from build123d import *

# Parameters (mm, degrees)
BOSS_EXTRU_1_DEPTH       = 320
BOSS_EXTRU_1_DEPTH_BACK  = 10
ESQUISSE3_W              = 200
ESQUISSE3_H              = 6
BOSS_EXTRU_2_DEPTH       = 56.1
ESQUISSE41_W             = 200
ESQUISSE41_H             = 330
BOSS_EXTRU_9_DEPTH       = 3
ENL_V_MAT_EXTRU_22_DEPTH = 6
CONG_8_R                 = 10
CONG_9_R                 = 16
ESQUISSE48_W             = 3
ESQUISSE48_H             = 2.4


with BuildPart() as part:
    # Esquisse1 → Boss.-Extru.1 (new body, two sides)
    with BuildSketch(Plane.XY) as boss_extru_1_sk:
        with BuildLine():
            Line((-95, 2), (95, 2))
            ThreePointArc((95, 2), (97.121320344, 2.878679656), (98, 5))
            Line((98, 5), (98, 17))
            ThreePointArc((98, 17), (99.464466094, 20.535533906), (103, 22))
            Line((103, 22), (127, 22))
            Line((127, 22), (132, 22))
            Line((132, 22), (132, 20))
            Line((132, 20), (127, 20))
            Line((127, 20), (103, 20))
            ThreePointArc((103, 20), (100.878679656, 19.121320344), (100, 17))
            Line((100, 17), (100, 0))
            Line((100, 0), (-100, 0))
            Line((-100, 0), (-100, 17))
            ThreePointArc((-100, 17), (-100.878679656, 19.121320344), (-103, 20))
            Line((-103, 20), (-127, 20))
            Line((-127, 20), (-132, 20))
            Line((-132, 20), (-132, 22))
            Line((-132, 22), (-127, 22))
            Line((-127, 22), (-103, 22))
            ThreePointArc((-103, 22), (-99.464466094, 20.535533906), (-98, 17))
            Line((-98, 17), (-98, 5))
            ThreePointArc((-98, 5), (-97.121320344, 2.878679656), (-95, 2))
        make_face()
    extrude(amount=BOSS_EXTRU_1_DEPTH)
    extrude(boss_extru_1_sk.sketch, amount=-BOSS_EXTRU_1_DEPTH_BACK)

    # Esquisse3 → Boss.-Extru.2 (add)
    with BuildSketch(Plane(origin=(0, 0, 0), x_dir=(-1, 0, 0), z_dir=(0, -1, 0))):
        with Locations((0, -317)):
            Rectangle(ESQUISSE3_W, ESQUISSE3_H)
    extrude(amount=BOSS_EXTRU_2_DEPTH)

    # Esquisse41 → Boss.-Extru.9 (add)
    with BuildSketch(Plane.XZ):
        with Locations((0, 155)):
            Rectangle(ESQUISSE41_W, ESQUISSE41_H)
        with BuildLine():
            Line((84, 314), (-84, 314))
            ThreePointArc((-84, 314), (-91.071067812, 311.071067812), (-94, 304))
            Line((-94, 304), (-94, 6))
            ThreePointArc((-94, 6), (-91.071067812, -1.071067812), (-84, -4))
            Line((-84, -4), (84, -4))
            ThreePointArc((84, -4), (91.071067812, -1.071067812), (94, 6))
            Line((94, 6), (94, 304))
            ThreePointArc((94, 304), (91.071067812, 311.071067812), (84, 314))
        make_face(mode=Mode.SUBTRACT)
    extrude(amount=BOSS_EXTRU_9_DEPTH)

    # Esquisse24 → Enlèv. mat.-Extru.22 (cut)
    with BuildSketch(Plane.XY.offset(320)):
        Polygon((65.886245289, -3), (56.523282614, -56.1), (100, -56.1), (100, -3), align=None)
        Polygon((-65.886245289, -3), (-56.523282614, -56.1), (-100, -56.1), (-100, -3), align=None)
    extrude(amount=-ENL_V_MAT_EXTRU_22_DEPTH, mode=Mode.SUBTRACT)

    # Congé8
    cong_8_edges = [part.edges().sort_by_distance(p)[0] for p in [
        (56.523282614, -56.1, 317),
        (-56.523282614, -56.1, 317),
    ]]
    fillet(cong_8_edges, radius=CONG_8_R)

    # Congé9
    cong_9_edges = [part.edges().sort_by_distance(p)[0] for p in [
        (65.886245289, -3, 317),
        (-65.886245289, -3, 317),
    ]]
    fillet(cong_9_edges, radius=CONG_9_R)

    # Enlèvement de matière-Balayage2: sweep along a curve in space
    with BuildLine() as enl_vement_de_mati_re_balayage2_path:
        Line((0, -3, -7), (84, -3, -7))
        ThreePointArc((84, -3, -7), (93.192388155, -3, -3.192388155), (97, -3, 6))
        Line((97, -3, 6), (97, -3, 304))
        ThreePointArc((97, -3, 304), (93.192388155, -3, 313.192388155), (84, -3, 317))
        Line((84, -3, 317), (79.311839388, -3, 317))
        ThreePointArc((63.55491534, -16.221629157, 317), (69.027237633, -6.74328891, 317), (79.311839388, -3, 317))
        Line((57.980363832, -47.836481777, 317), (63.55491534, -16.221629157, 317))
        ThreePointArc((48.132286302, -56.1, 317), (54.560162399, -53.760444431, 317), (57.980363832, -47.836481777, 317))
        Line((0, -56.1, 317), (48.132286302, -56.1, 317))
    # Esquisse48 → Enlèvement de matière-Balayage2 (sweep, cut)
    with BuildSketch(Plane(origin=(0, 0, 0), x_dir=(0, 0, -1), z_dir=(1, 0, 0))):
        with Locations((7, -1.8)):
            Rectangle(ESQUISSE48_W, ESQUISSE48_H)
    sweep(path=enl_vement_de_mati_re_balayage2_path.line, mode=Mode.SUBTRACT)


solid = part.part
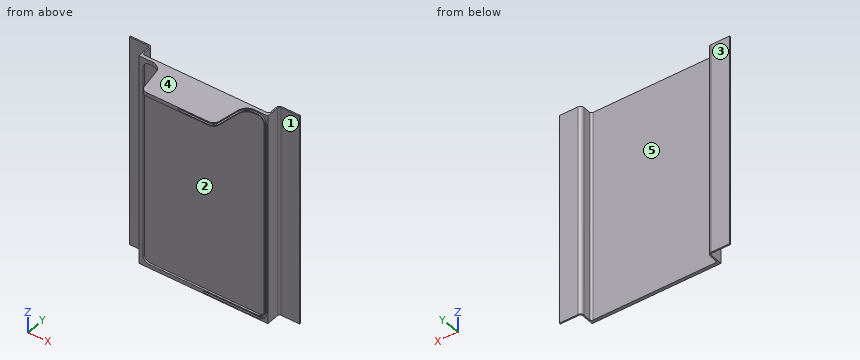
Design review of the part built by this model. Coordinates are the model's own, in mm. Face numbers are marked on the shaded views. A direction names the side the tool comes from. Coordinates: 2 decimals unless noted, no trailing zeros. Write each loop counter-clockwise with the first axis right and the second up, starting at its lowest first coordinate (ties: lowest second). Pieces come first, ordered by that corner, then holes. Notation, with made-up numbers: (52, 39.5) -> (76, 39.5) arc R19 ccw to (76, 44.5) -> close; hole circle Ø5 at (5, 57.25). An arc over 180 degrees is marked (long way). Write each question's results on one line, items separated by ' | '. Start each with the question number.
(1) Clearance check with flat-ended pins moving along their axes: P1, Ø1.5, axis at x = 21.5, z = 317.5, coming from the -Y side; P2, Ø3, axis at x = 44.5, z = 267.5, coming from the +Y side; P3, Ø16.5, axis at x = 44.5, y = -27.5, coming from the -Z side. State where each tip first meets the part, or that it passes through.
(2) Take a section at B-B on z = 112. Write out the cut boundary in (x, y).
(3) Take a section at C-C on x = 88. Write out the cut boundary in (y, z), and give its area (3 significant figures).
(4) Take a section at D-D on y = -38. Write out the cut boundary in (x, z), and give its area (3 significant figures).
(5) The part is to be moulded in two halves that separate along X. For the marked faces 4 and 5, say which applies: pulls with the +X half, pulls with the -X half, needs draft (parallel to the pull), parting line crosses it, or undercut.
(6) Take a section at A-A on y = 13. Write out the cut boundary in (x, z), and give its area (3 significant figures).
(7) Tool access review of the marked faces 1, 2 and 3: name each direction out of +Z, -Z, +X, -X, +Y, -Y from which nothing blocks a thin tool from reaching the whole face with its end or side.
(8) For line 1 along X through (y, z) = (-1.5, 302.5); line 2 along X through (y, z) = (13, 295); line 3 along Y through (x, z) = (116, 82.5), list the stretches that pass through material, from the lowest coordinate up. Write a range as from..to.
Results found:
1) P1: stops at y = -53.7 | P2: stops at y = 2 | P3: stops at z = 314
2) outline: (-132, 20) -> (-103, 20) arc R3 cw to (-100, 17) -> (-100, -3) -> (-94, -3) -> (-94, 0) -> (94, 0) -> (94, -3) -> (95.5, -3) -> (95.5, -0.6) -> (98.5, -0.6) -> (98.5, -3) -> (100, -3) -> (100, 17) arc R3 cw to (103, 20) -> (132, 20) -> (132, 22) -> (103, 22) arc R5 ccw to (98, 17) -> (98, 5) arc R3 cw to (95, 2) -> (-95, 2) arc R3 cw to (-98, 5) -> (-98, 17) arc R5 ccw to (-103, 22) -> (-132, 22) -> close
3) outline: (-3, -10) -> (2, -10) -> (2, 320) -> (-3, 320) -> (-3, 317.94) -> (-0.6, 317.94) -> (-0.6, 314.78) -> (-3, 314.78) -> (-3, 313.17) -> (0, 313.17) -> (0, -3.17) -> (-3, -3.17) -> (-3, -4.78) -> (-0.6, -4.78) -> (-0.6, -7.94) -> (-3, -7.94) -> close | area: 686 mm2
4) outline: (-59.71, 314) -> (59.71, 314) -> (59.71, 315.5) -> (57.28, 315.5) -> (57.28, 318.5) -> (59.71, 318.5) -> (59.71, 320) -> (-59.71, 320) -> close | area: 709 mm2
5) face 4: needs draft | face 5: undercut
6) outline: (-100, -10) -> (-98, -10) -> (-98, 320) -> (-100, 320) -> close; (98, -10) -> (100, -10) -> (100, 320) -> (98, 320) -> close | area: 1,320 mm2
7) face 1: +Z, -Z, +X, -Y | face 2: -Y | face 3: +Z, -Z, +X, -X, +Y
8) line 1: x = -100..-94, 94..95.5, 98.5..100 | line 2: x = -100..-98, 98..100 | line 3: y = 20..22
